For this review, take the finished solid that the model builds, in its own axes (mm). A direction names the side the tool comes from. Give positions to 0.01 mm unless a question says otherwise; leave off trailing zeros. Order: outer loops, then holes, each group sorted by start corner. A loop starts at its lowest first (then second) coordinate and runs counter-clockwise, first axis right, second up.
Item 1: For probe 1 along Y at (x, z) = (11.25, 21.5); probe 2 along X at (y, z) = (2.25, 25); probe 3 along Y at (x, z) = (11.25, 11.25), list the stretches that pass through material, from the lowest coordinate up.
Item 2: For P1, Ø3, axis at x = 16.5, z = 23.5, coming from the +Y side; P2, Ø1, axis at y = 4.5, z = 25.5, coming from the -X side; P3, Ø8, axis at x = 14.5, z = 26, coming from the +Y side; P4, Ø1.8, axis at x = 15, z = 25, coming from the +Y side, all flat-tipped, find the tip position at first contact; note any pin that passes through.
Item 3: Consider section B-B (x = 15). Give the boundary of the cut face in (y, z).
Item 4: Consider section C-C (z = 20.75). Give the boundary of the cut face in (x, y), plus the area to 3 significant figures.
Item 5: Consider section A-A (z = 25). Give the boundary of the cut face in (x, y).
Item 6: Consider section D-D (x = 11). Give the boundary of the cut face in (y, z), plus the area to 3 significant figures.
Item 7: The part is to be moulded in two halves that separate along X. For faces 1 (the cylindrical face through (7.473, 14.765, 5.451)), 2 (the flat face through (8, 3, 30)), 3 (the cylindrical face through (7.56, 5.25, 25.07)), say which applies: released by +X, released by -X, zero draft, split by the parting line, or undercut.
Item 8: Machinability: for faces 4 (the cylindrical face through (7.01, 13.48, 26.5)), 5 (the flat face through (12, 9, 10)), 6 (the flat face through (12, 9, 20)), which of the approach directions +Z, -Z, +X, -X, +Y, -Y give a long, thin tool a straight path to every point of the face, cutting with its end or side? Answer none if there is none.
```python
from build123d import *

# Parameters (mm, degrees)
EXTRUDE_1_DEPTH     = 30
SKETCH_2_R          = 1.5
CUT_EXTRUDE_1_DEPTH = 5
RIB_11_REACH        = 33.276
SKETCH_3_WALL_W     = 80.94250335
SKETCH_3_WALL_H     = 10
FILLET_1_R          = 3


with BuildPart() as part:
    # 草图1 → 凸台-拉伸1 (new body)
    with BuildSketch(Plane.XY):
        Polygon((0, 0), (20, 0), (20, 4), (5.712592027, 4), (10.59917335, 17.425771842), (6.840402867, 18.793852416), align=None)
    extrude(amount=EXTRUDE_1_DEPTH)

    # 草图2 → 切除-拉伸1 (cut)
    with BuildSketch(Plane.XZ):
        with Locations(Location((15, 25, 0), (0, 0, 270))):
            Circle(SKETCH_2_R)
        with Locations((15, 5)):
            Circle(SKETCH_2_R)
    cut_extrude_1 = extrude(amount=-CUT_EXTRUDE_1_DEPTH, mode=Mode.SUBTRACT)

    # 镜向1: 切除-拉伸1 across plane
    add(cut_extrude_1.mirror(Plane(origin=(0, 0, 0), x_dir=(0, 0, 1), z_dir=(-0.5735764363510445, 0.8191520442889929, 0))), mode=Mode.SUBTRACT)

    # 草图3 wall → 筋11 (add, up to next)
    with BuildSketch(Plane(origin=(15.299586675, 10.712885921, 15), x_dir=(0.573576436349, -0.81915204429, 0), z_dir=(0.81915204429, 0.573576436349, 0)), mode=Mode.PRIVATE) as rib_11_sk1:
        Rectangle(SKETCH_3_WALL_W, SKETCH_3_WALL_H)
    rib_11_tool1 = extrude(rib_11_sk1.sketch, amount=-RIB_11_REACH, mode=Mode.PRIVATE) - part.part
    add(rib_11_tool1.solids().sort_by_distance((15.299586675, 10.712885921, 15))[0])

    # 圆角1
    fillet_1_edges = [part.edges().sort_by_distance(p)[0] for p in [
        (5.712592027, 4, 25),
        (5.712592027, 4, 5),
    ]]
    fillet(fillet_1_edges, radius=FILLET_1_R)


solid = part.part
```
Resolved:
1. probe 1: y = 0 to 4
1. probe 2: x = 0.82 to 13.5, 16.5 to 20
1. probe 3: y = 0 to 16.5
2. P1: stops at y = 4
2. P2: stops at x = 1.46
2. P3: stops at y = 17.46
2. P4: passes through
3. outline: (0, 0) - (4, 0) - (4, 3.5) - (0, 3.5) - close; (0, 6.5) - (4, 6.5) - (4, 10) - (11.14, 10) - (11.14, 20) - (4, 20) - (4, 23.5) - (0, 23.5) - close; (0, 26.5) - (4, 26.5) - (4, 30) - (0, 30) - close
4. outline: (0, 0) - (20, 0) - (20, 4) - (10, 4) arc R3 cw to (7.18, 8.03) - (10.6, 17.43) - (6.84, 18.79) - close
4. area: 141 mm2
5. outline: (0, 0) - (13.5, 0) - (13.5, 4) - (10, 4) arc R3 cw to (7.18, 8.03) - (8.38, 11.32) - (4.62, 12.69) - close; (5.64, 15.5) - (9.4, 14.14) - (10.6, 17.43) - (6.84, 18.79) - close; (16.5, 0) - (20, 0) - (20, 4) - (16.5, 4) - close
6. outline: (0, 0) - (4, 0) - (4, 10) - (16.85, 10) - (16.85, 20) - (4, 20) - (4, 30) - (0, 30) - close
6. area: 249 mm2
7. face 1: undercut
7. face 2: zero draft
7. face 3: released by +X
8. face 4: none
8. face 5: -Z, +X
8. face 6: +Z, +X
